Here's how the part is built. I have some questions about the finished solid (model axes, mm). A direction names the side the tool comes from. Round coordinates to 2 decimals unless told otherwise and drop trailing zeros. Write each loop counter-clockwise with the first axis right and the second up, starting at its lowest first coordinate (ties: lowest second). Pieces come first, ordered by that corner, then holes. Notation, with made-up numbers: M -13,4.25 L -1,4.25 A32 ccw -1,42.25 Z; hole C 6,66.5 d7. An arc over 180 degrees is marked long. Use one line per item in the form item = value. Start each with the question number.
Q1. I want a section at D-D on z = -5.25. List the corners of the cut face in (x, y) for me.
Q2. I'm going to push a flat-ended pin straight in: pin 1 Ø7.5 at (x, z) = (-13, 1) entering from -Y. Where does the tip first touch, or does it pass through?
Q3. I want a section at B-B on x = -10.5. List the corners of the cut face in (y, z) for me.
Q4. We'd pull the mould along Z, two halves only. Please class faces 1 (the face through (-6.208, -1.521, 1.352)), 2 (the face through (-1, -4, -12.5)), 3 (the face through (-45, -4, 0)): +Z half, -Z half, draft (parallel to the pull), parting line (faces both ways), or undercut.
Q5. I want a section at C-C on z = 0. List the corners of the cut face in (x, y) for me.
Q6. For faces 4 (the face through (-43, -6, 0)), 5 (the face through (-1, -8, 0)), which set-ups out of +Z, -Z, +X, -X, +Y, -Y let a thin tool reach every point of the face, with its end or its side?
Q7. I want a section at A-A on y = -7. List the corners of the cut face in (x, z) for me, and give its area (3 significant figures).
Q8. I need wall thicknesses on line 1 along X through (y, z) = (-3.25, -3.25); line 2 along X through (y, z) = (-6.25, -6.5); line 3 along Z through (x, y) = (-35.5, -4.35). Which ranges of each line are inside material? Lowest first, please. Write a range as from..to.
```python
from build123d import *

# Parameters (mm, degrees)
F0_W     = 90
F0_H     = 25
F1_DEPTH = 8
F2_R     = 4.5
F2_R_2   = 7.75
F3_DEPTH = 8
F2_R_3   = 7.5
F4_DEPTH = 5


with BuildPart() as f1:
    # F0 (on Front) → F1 (new body)
    with BuildSketch(Plane.XZ):
        Rectangle(F0_W, F0_H)
    extrude(amount=F1_DEPTH)

    # F2 (on face) → F3 (cut, through all)
    with BuildSketch(Plane.XZ.offset(8)):
        with Locations((-35.5, 0)):
            Circle(F2_R)
        with Locations((-10.5, 0)):
            Circle(F2_R)
        with Locations((27, 0)):
            Circle(F2_R_2)
    extrude(amount=-F3_DEPTH, mode=Mode.SUBTRACT)

    # F2 (on face) → F4 (cut)
    with BuildSketch(Plane.XZ.offset(8)):
        with Locations((-35.5, 0)):
            Circle(F2_R_3)
        with Locations((-35.5, 0)):
            Circle(F2_R, mode=Mode.SUBTRACT)
        with Locations((-10.5, 0)):
            Circle(F2_R_3)
        with Locations((-10.5, 0)):
            Circle(F2_R, mode=Mode.SUBTRACT)
        with Locations((27, 0)):
            Circle(F2_R_2)
    extrude(amount=-F4_DEPTH, mode=Mode.SUBTRACT)


solid = f1.part
```
Reported:
q1.outline = M -45,-8 L -40.86,-8 L -40.86,-3 L -30.14,-3 L -30.14,-8 L -15.86,-8 L -15.86,-3 L -5.14,-3 L -5.14,-8 L 21.3,-8 L 21.3,0 L -45,0 Z; M 32.7,-8 L 45,-8 L 45,0 L 32.7,0 Z
q2.pin_1 = -3
q3.outline = M -8,-12.5 L 0,-12.5 L 0,-4.5 L -3,-4.5 L -3,-7.5 L -8,-7.5 Z; M -8,7.5 L -3,7.5 L -3,4.5 L 0,4.5 L 0,12.5 L -8,12.5 Z
q4.face_1 = undercut
q4.face_2 = -Z half
q4.face_3 = draft
q5.outline = M -45,-8 L -43,-8 L -43,-3 L -40,-3 L -40,0 L -45,0 Z; M -31,-3 L -28,-3 L -28,-8 L -18,-8 L -18,-3 L -15,-3 L -15,0 L -31,0 Z; M -6,-3 L -3,-3 L -3,-8 L 19.25,-8 L 19.25,0 L -6,0 Z; M 34.75,-8 L 45,-8 L 45,0 L 34.75,0 Z
q6.face_4 = -Y
q6.face_5 = +Z, -Z, +X, -X, -Y
q7.outline = M -45,-12.5 L 45,-12.5 L 45,12.5 L -45,12.5 Z; hole C -35.5,0 d15; hole C -10.5,0 d15; hole C 27,0 d15.5
q7.area = 1,710 mm^2
q8.line_1 = -45..-42.26, -28.74..-17.26, -3.74..19.96, 34.04..45
q8.line_2 = -45..-39.24, -31.76..-14.24, -6.76..22.78, 31.22..45
q8.line_3 = -12.5..-7.5, 7.5..12.5
